```python
from build123d import *

# Parameters (mm, degrees)
SKETCH1_W                = 30
SKETCH1_H                = 110
BOSS_EXTRUDE1_DEPTH      = 20
CUT_EXTRUDE1_DEPTH       = 60
CHAMFER1_SIZE            = 8
BOSS_EXTRUDE2_DEPTH      = 21
BOSS_EXTRUDE3_DEPTH      = 50
BOSS_EXTRUDE3_DEPTH_BACK = 18
CUT_EXTRUDE3_DEPTH       = 260
SHELL1_START             = 3
SHELL1_DEPTH             = 17
SHELL1_START_2           = -47
SHELL1_2_DEPTH           = 50
SHELL1_START_3           = 2
SHELL1_3_DEPTH           = 1


# Read off the part's stored shape, not the designer's step: Shell1
with BuildPart() as part:
    # Sketch1 → Boss-Extrude1 (new body)
    with BuildSketch(Plane.XY):
        with Locations((15, 55)):
            Rectangle(SKETCH1_W, SKETCH1_H)
    extrude(amount=BOSS_EXTRUDE1_DEPTH)

    # Sketch2 → Cut-Extrude1 (cut)
    with BuildSketch(Plane.XY.offset(20)):
        Polygon((25, 95.443111243), (20, 104.103365281), (10, 104.103365281), (5, 95.443111243), (10, 86.782857205), (20, 86.782857205), align=None)
    extrude(amount=-CUT_EXTRUDE1_DEPTH, mode=Mode.SUBTRACT)

    # Chamfer1
    chamfer1_edges = [part.edges().sort_by_distance(p)[0] for p in [
        (0, 110, 10),
        (30, 110, 10),
    ]]
    chamfer(chamfer1_edges, length=CHAMFER1_SIZE)

    # Sketch3 → Boss-Extrude2 (add)
    with BuildSketch(Plane.XY.offset(20)):
        Polygon((-40.427156972, -1.878677735), (-53.835121548, -1.878677735), (0, 102), (0, 76.128383271), align=None)
        Polygon((30, 102), (83.835121548, -1.878677735), (70.427156972, -1.878677735), (30, 76.128383271), align=None)
    extrude(amount=-BOSS_EXTRUDE2_DEPTH)

    # Sketch5 → Boss-Extrude3 (add, two sides: drawn at the far end of the back side and taken through both)
    with BuildSketch(Plane(origin=(0, 0, 0), x_dir=(-1, 0, 0), z_dir=(0, 0, -1)).offset(-BOSS_EXTRUDE3_DEPTH_BACK)):
        Polygon((-83.835121548, -1.878677735), (-71.933606609, 21.086137785), (-50.213578486, 37.124852768), (-70.427156972, -1.878677735), align=None)
        Polygon((40.427156972, -1.878677735), (53.835121548, -1.878677735), (41.933606609, 21.086137785), (20.213578486, 37.124852768), align=None)
    extrude(amount=BOSS_EXTRUDE3_DEPTH + BOSS_EXTRUDE3_DEPTH_BACK)

    # Sketch8 → Cut-Extrude3 (cut)
    with BuildSketch(Plane.XY.offset(20)):
        with BuildLine():
            Line((0, 76.128383271), (0, -18.897317389))
            Line((0, -18.897317389), (30, -18.897317389))
            Line((30, -18.897317389), (30, 76.128383271))
            ThreePointArc((30, 76.128383271), (15, 70.851219372), (0, 76.128383271))
        make_face()
    extrude(amount=-CUT_EXTRUDE3_DEPTH, mode=Mode.SUBTRACT)

    # Shell1 outline → Shell1 (cut)
    with BuildSketch(Plane.XY.offset(SHELL1_START)):
        with BuildLine():
            Line((28.464101615, 95.443111243), (21.732050808, 83.782857205))
            Line((21.732050808, 83.782857205), (8.267949192, 83.782857205))
            Line((8.267949192, 83.782857205), (1.535898385, 95.443111243))
            Line((1.535898385, 95.443111243), (6.795296251, 104.552655563))
            Line((6.795296251, 104.552655563), (2.449804376, 100.207163689))
            Line((2.449804376, 100.207163689), (-48.901429901, 1.121322265))
            Line((-48.901429901, 1.121322265), (-42.251348803, 1.121322265))
            Line((-42.251348803, 1.121322265), (-0.820872426, 81.064359083))
            ThreePointArc((-0.820872426, 81.064359083), (15, 73.851219372), (30.820872426, 81.064359083))
            Line((30.820872426, 81.064359083), (72.251348803, 1.121322265))
            Line((72.251348803, 1.121322265), (78.901429901, 1.121322265))
            Line((78.901429901, 1.121322265), (27.550195624, 100.207163689))
            Line((27.550195624, 100.207163689), (23.204703749, 104.552655563))
            Line((23.204703749, 104.552655563), (28.464101615, 95.443111243))
        make_face()
    extrude(amount=SHELL1_DEPTH, mode=Mode.SUBTRACT)

    # Shell1 2 outline → Shell1 2 (cut)
    with BuildSketch(Plane.XY.offset(SHELL1_START_2)):
        Polygon((78.901429901, 1.121322265), (69.590785527, 19.086869637), (58.818087877, 27.041750092), (72.251348803, 1.121322265), align=None)
        Polygon((-28.818087877, 27.041750092), (-39.590785527, 19.086869637), (-48.901429901, 1.121322265), (-42.251348803, 1.121322265), align=None)
    extrude(amount=SHELL1_2_DEPTH, mode=Mode.SUBTRACT)

    # Shell1 3 outline → Shell1 3 (cut)
    with BuildSketch(Plane.XY.offset(SHELL1_START_3)):
        Polygon((69.590785527, 19.086869637), (33, 89.691380382), (33, 76.85957818), (58.818087877, 27.041750092), align=None)
        Polygon((-3, 76.85957818), (-3, 89.691380382), (-39.590785527, 19.086869637), (-28.818087877, 27.041750092), align=None)
    extrude(amount=SHELL1_3_DEPTH, mode=Mode.SUBTRACT)


solid = part.part
```
Work out the finished part from the listing and answer in its coordinate system (mm). A direction names the side the tool comes from. Give positions to 0.01 mm unless a question says otherwise; leave off trailing zeros. Loops run counter-clockwise (first coordinate to the right, second up) from the corner with the lowest first, then second, coordinate; pieces in that order, holes last. Notation, with made-up numbers: (6.5, 18) -> (56.5, 18) arc R11 cw to (56.5, 39) -> close; hole circle Ø4 at (87.25, 46). An arc over 180 degrees is marked (long way). Use CSV: the item, a comma, the result in double quotes.
1. A tool of negligible diameter and unlimited length cuts with its end or side. For faces 4 (the flat face through (68, 13, -50)), 5 (the flat face through (-40, 12, -47)), 6 (the flat face through (7.465, 91.174, 10.14)), from which of +Z, -Z, +X, -X, +Y, -Y can it reach the whole face along a straight path? Write none if from no direction.
Found:
face 4,"-Z, +X, -X, +Y, -Y"
face 5,"+Z"
face 6,"+Z, -Z"
2. The part is cut by section A-A (z = -32). Write down the section's boundary in (x, y).
Found:
outline,"(-53.84, -1.88) -> (-40.43, -1.88) -> (-20.21, 37.12) -> (-41.93, 21.09) -> close; (50.21, 37.12) -> (70.43, -1.88) -> (83.84, -1.88) -> (71.93, 21.09) -> close; hole (-48.9, 1.12) -> (-42.25, 1.12) -> (-28.82, 27.04) -> (-39.59, 19.09) -> close; hole (58.82, 27.04) -> (72.25, 1.12) -> (78.9, 1.12) -> (69.59, 19.09) -> close"
3. The mould has two halves that part along X. Classify faces 1 (the flat face through (61.23, 28.99, -25.16)), 2 (the flat face through (7.535, 99.834, 10.14)), 3 (the flat face through (46, 62, -1)): +X half, -X half, draft (parallel to the pull), parting line (faces both ways), or undercut.
Found:
face 1,"+X half"
face 2,"undercut"
face 3,"draft"
4. The part is cut by section D-D (x = 16). Write down the section's boundary in (y, z), then the cut area to 3 significant figures.
Found:
outline,"(70.87, 0) -> (86.78, 0) -> (86.78, 20) -> (83.78, 20) -> (83.78, 3) -> (73.88, 3) -> (73.88, 20) -> (70.87, 20) -> close; (104.1, 0) -> (110, 0) -> (110, 20) -> (104.1, 20) -> close"
area,"268 mm^2"
5. Flat-ended cylindrical pins translate along their axes: pin 1 Ø1.1 at (y, z) = (84, 2.5) entering from -X; pin 2 Ø15 at (x, y) = (18, 88) entering from -Z; pin 3 Ø5.5 at (x, z) = (74.5, -11.5) entering from +Y. Find the tip coordinate at first contact, or state that the pin passes through.
Found:
pin 1,"x = -9.61"
pin 2,"z = 0"
pin 3,"y = 21.22"
6. Straight lines are drawn through the part: line 1 (Y direction, x = 18.5, z = 9); line 2 (X direction, y = 16, z = -24); line 3 (Y direction, x = 11, z = 14). For each, find the intervals that lie inside material, in ascending order.
Found:
line 1,"71.11 to 74.15, 83.78 to 86.78, 104.1 to 110"
line 2,"-44.57 to -41.19, -34.54 to -31.16, 61.16 to 64.54, 71.19 to 74.57"
line 3,"71.19 to 74.24, 83.78 to 86.78, 104.1 to 110"
7. The part is cut by section B-B (y = 8.5). Write down the section's boundary in (x, z), then the cut area to 3 significant figures.
Found:
outline,"(-48.46, -50) -> (-35.05, -50) -> (-35.05, 20) -> (-38.43, 20) -> (-38.43, -47) -> (-45.08, -47) -> (-45.08, 20) -> (-48.46, 20) -> close; (65.05, -50) -> (78.46, -50) -> (78.46, 20) -> (75.08, 20) -> (75.08, -47) -> (68.43, -47) -> (68.43, 20) -> (65.05, 20) -> close"
area,"986 mm^2"
8. The part is cut by section C-C (z = 11.5). State how many separate pieces and enclosed holes the cut face has, then the cut area to 3 significant figures.
Found:
separate pieces,"1"
enclosed holes,"2"
area,"1,690 mm^2"
